CAD build for the part. Positions are in the model's coordinates, mm. Face numbers are marked on the shaded views. A direction names the side the tool comes from. Coordinates: 2 decimals unless noted, no trailing zeros. Order: outer loops, then holes, each group sorted by start corner. A loop starts at its lowest first (then second) coordinate and runs counter-clockwise, first axis right, second up. Notation, with made-up numbers: M -19.5,-7 L 29.5,-7 A14 ccw 29.5,-2 Z; hole C 15.5,-21.5 d8. An arc over 180 degrees is marked long. Write item = value, one per line.
from build123d import *

# Parameters (mm, degrees)
SKETCH1_W               = 30
SKETCH1_H               = 60
SKETCH1_R               = 2.9
BOSS_EXTRUDE1_DEPTH     = 3
SKETCH2_W               = 3
SKETCH2_H               = 60
BOSS_EXTRUDE2_DEPTH     = 65
SKETCH5_W               = 7
SKETCH5_H               = 20
BOSS_EXTRUDE3_DEPTH     = 60
CUT_EXTRUDE1_REACH      = 32
SKETCH3_R               = 1.5
SKETCH3_R_2             = 6
SKETCH3_R_3             = 2
SKETCH4_R               = 1.5
SKETCH4_R_2             = 6
CUT_EXTRUDE2_DEPTH      = 28
CUT_EXTRUDE2_DEPTH_BACK = 4


with BuildPart() as part:
    # Sketch1 → Boss-Extrude1 (new body)
    with BuildSketch(Plane.XY):
        Rectangle(SKETCH1_W, SKETCH1_H)
        with Locations((0, 15)):
            Circle(SKETCH1_R, mode=Mode.SUBTRACT)
        with Locations((0, -15)):
            Circle(SKETCH1_R, mode=Mode.SUBTRACT)
    extrude(amount=BOSS_EXTRUDE1_DEPTH)

    # Sketch2 → Boss-Extrude2 (add)
    with BuildSketch(Plane.XY.offset(3)):
        with Locations((-13.5, 0)):
            Rectangle(SKETCH2_W, SKETCH2_H)
        with Locations((13.5, 0)):
            Rectangle(SKETCH2_W, SKETCH2_H)
    extrude(amount=BOSS_EXTRUDE2_DEPTH)

    # Sketch5 → Boss-Extrude3 (add)
    with BuildSketch(Plane(origin=(0, 30, 0), x_dir=(1, 0, 0), z_dir=(0, 1, 0))):
        with Locations((8.5, -16.320138996)):
            Rectangle(SKETCH5_W, SKETCH5_H)
        with Locations((-8.5, -16.320138996)):
            Rectangle(SKETCH5_W, SKETCH5_H)
    extrude(amount=-BOSS_EXTRUDE3_DEPTH)

    # Sketch3 → Cut-Extrude1 (cut, up to next)
    with BuildSketch(Plane.ZY.offset(15), mode=Mode.PRIVATE) as cut_extrude1_sk1:
        with Locations((13, 20)):
            Circle(SKETCH3_R)
    cut_extrude1_tool1 = extrude(cut_extrude1_sk1.sketch, amount=-CUT_EXTRUDE1_REACH, mode=Mode.PRIVATE) & part.part
    add(cut_extrude1_tool1.solids().sort_by_distance((-15, 20, 13))[0], mode=Mode.SUBTRACT)
    # Sketch3 → Cut-Extrude1 (cut, up to next)
    with BuildSketch(Plane.ZY.offset(15), mode=Mode.PRIVATE) as cut_extrude1_sk2:
        with Locations((38, 0)):
            Circle(SKETCH3_R_2)
    cut_extrude1_tool2 = extrude(cut_extrude1_sk2.sketch, amount=-CUT_EXTRUDE1_REACH, mode=Mode.PRIVATE) & part.part
    add(cut_extrude1_tool2.solids().sort_by_distance((-15, 0, 38))[0], mode=Mode.SUBTRACT)
    # Sketch3 → Cut-Extrude1 (cut, up to next)
    with BuildSketch(Plane.ZY.offset(15), mode=Mode.PRIVATE) as cut_extrude1_sk3:
        with Locations((20.25, 0)):
            Circle(SKETCH3_R_3)
    cut_extrude1_tool3 = extrude(cut_extrude1_sk3.sketch, amount=-CUT_EXTRUDE1_REACH, mode=Mode.PRIVATE) & part.part
    add(cut_extrude1_tool3.solids().sort_by_distance((-15, 0, 20.25))[0], mode=Mode.SUBTRACT)
    # Sketch3 → Cut-Extrude1 (cut, up to next)
    with BuildSketch(Plane.ZY.offset(15), mode=Mode.PRIVATE) as cut_extrude1_sk4:
        with Locations((38, 17.75)):
            Circle(SKETCH3_R_3)
    cut_extrude1_tool4 = extrude(cut_extrude1_sk4.sketch, amount=-CUT_EXTRUDE1_REACH, mode=Mode.PRIVATE) & part.part
    add(cut_extrude1_tool4.solids().sort_by_distance((-15, 17.75, 38))[0], mode=Mode.SUBTRACT)
    # Sketch3 → Cut-Extrude1 (cut, up to next)
    with BuildSketch(Plane.ZY.offset(15), mode=Mode.PRIVATE) as cut_extrude1_sk5:
        with Locations((55.75, 0)):
            Circle(SKETCH3_R_3)
    cut_extrude1_tool5 = extrude(cut_extrude1_sk5.sketch, amount=-CUT_EXTRUDE1_REACH, mode=Mode.PRIVATE) & part.part
    add(cut_extrude1_tool5.solids().sort_by_distance((-15, 0, 55.75))[0], mode=Mode.SUBTRACT)
    # Sketch3 → Cut-Extrude1 (cut, up to next)
    with BuildSketch(Plane.ZY.offset(15), mode=Mode.PRIVATE) as cut_extrude1_sk6:
        with Locations((38, -17.75)):
            Circle(SKETCH3_R_3)
    cut_extrude1_tool6 = extrude(cut_extrude1_sk6.sketch, amount=-CUT_EXTRUDE1_REACH, mode=Mode.PRIVATE) & part.part
    add(cut_extrude1_tool6.solids().sort_by_distance((-15, -17.75, 38))[0], mode=Mode.SUBTRACT)
    # Sketch3 → Cut-Extrude1 (cut, up to next)
    with BuildSketch(Plane.ZY.offset(15), mode=Mode.PRIVATE) as cut_extrude1_sk7:
        with Locations((13, -20)):
            Circle(SKETCH3_R)
    cut_extrude1_tool7 = extrude(cut_extrude1_sk7.sketch, amount=-CUT_EXTRUDE1_REACH, mode=Mode.PRIVATE) & part.part
    add(cut_extrude1_tool7.solids().sort_by_distance((-15, -20, 13))[0], mode=Mode.SUBTRACT)

    # Sketch4 → Cut-Extrude2 (cut, two sides)
    with BuildSketch(Plane.ZY.offset(-12)) as cut_extrude2_sk:
        with Locations((13, -20)):
            Circle(SKETCH4_R)
        with Locations((13, 20)):
            Circle(SKETCH4_R)
        with Locations((38, 0)):
            Circle(SKETCH4_R_2)
    extrude(amount=CUT_EXTRUDE2_DEPTH, mode=Mode.SUBTRACT)
    extrude(cut_extrude2_sk.sketch, amount=-CUT_EXTRUDE2_DEPTH_BACK, mode=Mode.SUBTRACT)


solid = part.part
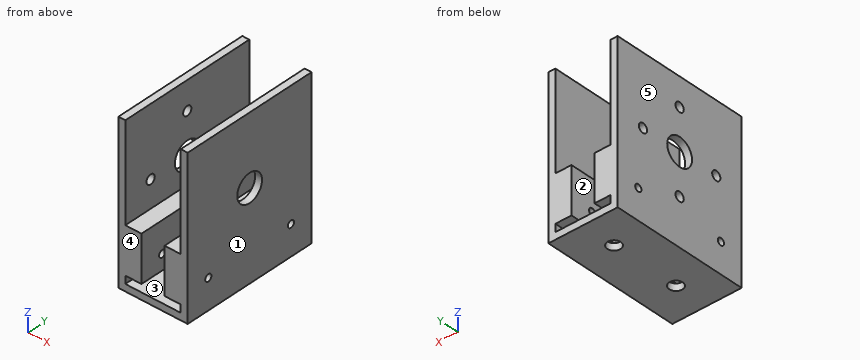
(1) Tool access for the marked faces 1 and 2: list every direction of +Z, -Z, +X, -X, +Y, -Y with a clear straight run to the whole face (end or side of a thin tool).
Evaluation:
face_1 = +Z, -Z, +X, +Y, -Y
face_2 = +Z, +Y, -Y
(2) Slice it at A-A, the plane x = 8.25. Write the cut outline in (y, z).
Evaluation:
outline = M -30,0 L 30,0 L 30,3 L -30,3 Z; M -30,6.32 L 30,6.32 L 30,26.32 L -30,26.32 Z; hole C -20,13 d3; hole C 20,13 d3
(3) Slice it at B-B, the plane z = 24.5. Write the cut outline in (x, y), then the cut area to 3 significant figures.
Evaluation:
outline = M -15,-30 L -5,-30 L -5,30 L -15,30 Z; M 5,-30 L 15,-30 L 15,30 L 5,30 Z
area = 1,200 mm²
(4) Pin check, flat tips, straight feed: pin 1 Ø9.5 at (y, z) = (0, 38) entering from -X; pin 2 Ø2 at (x, y) = (7, 3) entering from +Z. Stop position of each tip, or through.
Evaluation:
pin_1 = through
pin_2 = 26.32
(5) Pull direction X, two halves, no side cores. Call the marked faces 3, 4 and 5: +X half, -X half, draft (parallel to the pull), parting line (faces both ways), or undercut.
Evaluation:
face_3 = undercut
face_4 = draft
face_5 = -X half
(6) Slice it at C-C, the plane x = -8.5. Write the cut outline in (y, z).
Evaluation:
outline = M -30,0 L 30,0 L 30,3 L -30,3 Z; M -30,6.32 L 30,6.32 L 30,26.32 L -30,26.32 Z; hole C -20,13 d3; hole C 0,20.25 d4; hole C 20,13 d3
(7) Wall check: line 1 (Y direction, x = -7.5, z = 13); line 2 (Z direction, x = 11.5, y = 2); line 3 (X direction, y = -13.5, z = 33). Give the ranges that are in metal, low to high. Write a range as from..to.
Evaluation:
line_1 = -30..-21.5, -18.5..18.5, 21.5..30
line_2 = 0..3, 6.32..26.32
line_3 = -15..-12, 12..15
(8) Slice it at D-D, the plane z = 13. Write the cut outline in (x, y).
Evaluation:
outline = M -15,-30 L -5,-30 L -5,-21.5 L -15,-21.5 Z; M -15,-18.5 L -5,-18.5 L -5,18.5 L -15,18.5 Z; M -15,21.5 L -5,21.5 L -5,30 L -15,30 Z; M 5,-30 L 15,-30 L 15,-21.5 L 5,-21.5 Z; M 5,-18.5 L 15,-18.5 L 15,18.5 L 5,18.5 Z; M 5,21.5 L 15,21.5 L 15,30 L 5,30 Z
